Read the model definition and answer for the solid it produces. Units are mm, in the model's axes. Face numbers are marked on the shaded views. A direction names the side the tool comes from. Coordinates: 2 decimals unless noted, no trailing zeros. Loops run counter-clockwise (first coordinate to the right, second up) from the corner with the lowest first, then second, coordinate; pieces in that order, holes last. Notation, with made-up numbers: (33.5, 32.5) - (79.5, 32.5) arc R18 cw to (79.5, 58.5) - close; hole circle Ø7 at (-31.5, 30). An arc over 180 degrees is marked (long way). One line per question, with ' | ' between items. Start each with the question number.
Autodesk Inventor part; units mm, degrees
ref_plane "YZ Plane" through (0, 0, 0) normal (1, 0, 0) x (0, 1, 0)
ref_plane "XZ Plane" through (0, 0, 0) normal (0, 1, 0) x (-1, 0, 0)
ref_plane "XY Plane" through (0, 0, 0) normal (0, 0, 1) x (1, 0, 0)
sketch "Sketch1" plane through (0, 0, 0) normal (0, 0, 1) x (1, 0, 0)
  line L0 (-200, 100) -> (200, 100)
  line L1 (-200, -100) -> (-200, 100)
  line L2 (200, -100) -> (-200, -100)
  line L3 (200, 100) -> (200, -100)
  line L4 (-121, -18.2) -> (-94.2029, -18.2)
  line L5 (-94.2029, -18.2) -> (188.9125, -18.2)
  line L6 (110, -18.2) -> (70, -18.2)
  line L7 (70, -18.2) -> (150, -18.2)
  line L8 (150, -18.2) -> (150, -58.2)
  line L9 (150, -58.2) -> (70, -58.2)
  line L10 (70, -58.2) -> (70, -18.2)
  line L11 (150, -58.2) -> (145, -58.2)
  circle A0 centre (145, -53.2) radius 1.5
  circle A1 centre (145, -23.2) radius 1.5
  circle A2 centre (75, -23.2) radius 1.5
  circle A3 centre (75, -53.2) radius 1.5
  point P0 (0, 0)
  dimension "d2" = 80
  dimension "d3" = 40
  dimension "d4" = 5
extrude "Extrusion1" add sketch "Sketch1" along normal blind 3.7 contours L5 L8 L9 L10
ref_plane "Work Plane1" through (109.8736, -37.15, 11.15) normal (0, 1, 0) x (-1, 0, 0)
sketch "Sketch2" plane through (109.8736, -37.15, 11.15) normal (0, 1, 0) x (-1, 0, 0)
  line L0 (3.756, 7.45) -> (-3.756, 7.45)
  arc A0 (-6.6658, 7.3197) -> (-9.9, 0) centre (0, 0) ccw
  arc A1 (9.9, 0) -> (6.6658, 7.3197) centre (0, 0) ccw
  arc A2 (6.6658, 7.3197) -> (6.3291, 7.45) centre (6.3291, 6.95) ccw
  arc A3 (-6.3291, 7.45) -> (-6.6658, 7.3197) centre (-6.3291, 6.95) ccw
  line L1 (-3.756, 7.45) -> (-6.3291, 7.45)
  line L2 (6.3291, 7.45) -> (3.756, 7.45)
  arc A4 (-6.3291, 9.45) -> (-8.0124, 8.7984) centre (-6.3291, 6.95) ccw
  line L3 (-6.3291, 9.45) -> (-3.756, 9.45)
  line L4 (-3.756, 9.45) -> (3.756, 9.45)
  line L5 (3.756, 9.45) -> (6.3291, 9.45)
  arc A5 (8.0124, 8.7984) -> (6.3291, 9.45) centre (6.3291, 6.95) ccw
  line L6 (-11.9, 0) -> (-11.9, -5.45)
  line L7 (39.8736, -7.45) -> (-40.1264, -7.45)
  line L8 (-11.9, -7.45) -> (-21.9, -7.45)
  line L9 (-21.9, -7.45) -> (-21.9, -5.45)
  line L10 (-21.9, -5.45) -> (-11.9, -5.45)
  line L11 (11.9, -7.45) -> (21.9, -7.45)
  line L12 (21.9, -7.45) -> (21.9, -5.45)
  line L13 (21.9, -5.45) -> (11.9, -5.45)
  line L14 (9.9, 0) -> (9.9, -7.45)
  line L15 (-9.9, 0) -> (-9.9, -7.45)
  arc A6 (-8.0124, 8.7984) -> (-11.9, 0) centre (0, 0) ccw
  arc A7 (11.9, 0) -> (8.0124, 8.7984) centre (0, 0) ccw
  line L16 (11.9, 0) -> (11.9, -5.45)
  line L17 (-21.9, -7.45) -> (21.9, -7.45)
  point P0 (109.8736, -11.15)
  point P1 (21.9, -7.45)
  point P2 (-21.9, -7.45)
  dimension "d21" = 10
  dimension "d22" = 2
  dimension "d23" = 10
  dimension "d24" = 2
  dimension "d26" = 2
extrude "Extrusion2" add sketch "Sketch2" against normal blind 18 contours L0 L1 A3 A0 L15 L7 L9 L10 L6 A6 A4 L3 L4 L5 A5 A7 L16 L13 L12 L14 A1 A2 L2
sketch "Sketch3" plane through (121.7736, -37.15, 5.7) normal (0, 0, 1) x (1, 0, 0)
  line L0 (10, -18) -> (0, -18)
  circle A0 centre (5, -9) radius 1.5
  line L1 (-33.8, -18) -> (-33.8, 0)
  line L2 (-33.8, -18) -> (-33.8, -9)
  circle A1 centre (-28.8, -9) radius 1.5
  point P0 (-121.7736, 37.15)
hole "Hole1" at (126.7736, -46.15, 5.7) at (92.9736, -46.15, 5.7) direction (0, 0, -1) diameter 3 end through all
properties part number "suporte_motor_1"
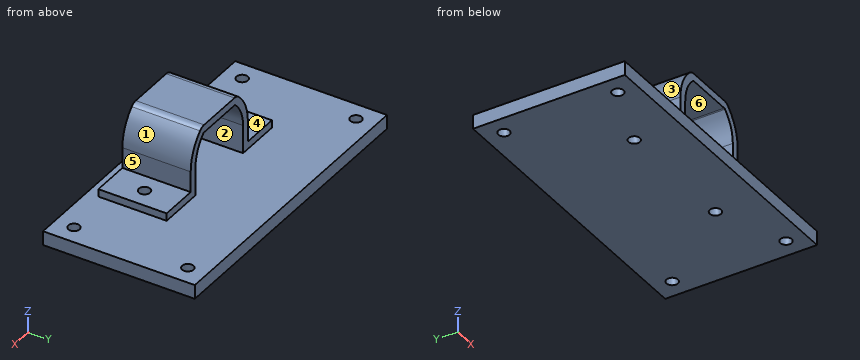
1) Which of the six approach directions +Z, -Z, +X, -X, +Y, -Y give full straight-line access (tool end or side, diameter ignored) to the marked faces 4, 5 and 6?
2) The part is cut by section C-C on z = 7.75. Write down the section's boundary in (x, y).
3) Given pin 1 Ø5 at (x, y) = (92.97, -46.15) entering from +Z; pin 2 Ø8 at (y, z) = (-49, 8) entering from -X; pin 3 Ø2 at (y, z) = (-34.5, 15) entering from -X; pin 4 Ø5 at (y, z) = (-54, 9) entering from -X, each flat-ended and moving along its own axis, determine where each tip first touches the part or whether it passes through.
4) Find the intervals of material crossed by line 1 along X through (y, z) = (-46.15, 3.95); line 2 along Y through (x, z) = (145, 1.75); line 3 along X through (y, z) = (-39, 8.75), in increasing order. Write a range as from..to.
5) The part is cut by section D-D on y = -23.2. Write down the section's boundary in (x, z), and give its area (3 significant figures).
6) The part is cut by section B-B on x = 75. Write down the section's boundary in (y, z).
7) The part is cut by section A-A on y = -53.2. Count the separate pieces of the cut face and the enclosed holes in it, and give its area (3 significant figures).
8) The mould has two halves that part along X. Classify the marked faces 1, 2 and 3: released by +X, released by -X, zero draft, split by the parting line, or undercut.
Answer below:
1) face 4: +Z, -X, +Y, -Y | face 5: +Z, +X, +Y, -Y | face 6: +Y, -Y
2) outline: (97.97, -55.15) - (99.97, -55.15) - (99.97, -37.15) - (97.97, -37.15) - close; (119.77, -55.15) - (121.77, -55.15) - (121.77, -37.15) - (119.77, -37.15) - close
3) pin 1: z = 5.7 | pin 2: x = 87.97 | pin 3: through | pin 4: x = 97.97
4) line 1: 87.97..91.47, 94.47..99.97, 119.77..125.27, 128.27..131.77 | line 2: -58.2..-54.7, -51.7..-24.7, -21.7..-18.2 | line 3: 97.97..99.97, 119.77..121.77
5) outline: (70, 0) - (73.5, 0) - (73.5, 3.7) - (70, 3.7) - close; (76.5, 0) - (143.5, 0) - (143.5, 3.7) - (76.5, 3.7) - close; (146.5, 0) - (150, 0) - (150, 3.7) - (146.5, 3.7) - close | area: 274 mm2
6) outline: (-58.2, 0) - (-54.7, 0) - (-54.7, 3.7) - (-58.2, 3.7) - close; (-51.7, 0) - (-24.7, 0) - (-24.7, 3.7) - (-51.7, 3.7) - close; (-21.7, 0) - (-18.2, 0) - (-18.2, 3.7) - (-21.7, 3.7) - close
7) separate pieces: 3 | enclosed holes: 1 | area: 410 mm2
8) face 1: released by +X | face 2: undercut | face 3: released by -X
